Autodesk Fusion 360 part; units mm, degrees
sketch "Esquisse1" plane through (0, 0, 0) normal (0, 0, 1) x (1, 0, 0)
  line L0 (7, 0) -> (13, 0)
  line L1 (20, 7) -> (20, 21)
  line L2 (13, 28) -> (7, 28)
  line L3 (0, 21) -> (0, 7)
  line L4 (10, 28) -> (10, 0) construction
  circle A0 centre (10, 23.45) radius 2.1
  circle A1 centre (10, 4.55) radius 2.1
  line L5 (-6, 20) -> (25, 20) construction
  line L6 (25, 20) -> (25, 8) construction
  line L7 (25, 8) -> (-6, 8) construction
  line L8 (-6, 8) -> (-6, 20) construction
  line L9 (13, 0) -> (20, 7)
  line L10 (7, 0) -> (0, 7)
  line L11 (20, 21) -> (13, 28)
  line L12 (7, 28) -> (0, 21)
  point P0 (20, 0)
  point P1 (20, 28)
  point P2 (0, 28)
  dimension "d1" = 20
  dimension "d2" = 28
  dimension "d3" = 4.2
  dimension "d4" = 4.2
  dimension "d5" = 18.9
  dimension "d6" = 4.55
  dimension "d7" = 12
  dimension "d8" = 8
  dimension "d9" = 7
  dimension "d10" = 7
  dimension "d11" = 7
  dimension "d12" = 7
  dimension "d13" = 7
  dimension "d14" = 7
  dimension "d15" = 7
  dimension "d16" = 7
extrude "Extrusion1" add sketch "Esquisse1" along normal blind 14
sketch "Esquisse2" plane through (20, 0, 0) normal (1, 0, 0) x (0, 1, 0)
  line L0 (7, 0) -> (21, 0)
  line L1 (21, 0) -> (21, 14)
  line L2 (21, 14) -> (7, 14)
  line L3 (7, 14) -> (7, 0)
  circle A0 centre (14, 15) radius 6
  dimension "d19" = 12
  dimension "d20" = 15
  dimension "d21" = 7
extrude "Extrusion2" cut sketch "Esquisse2" against normal blind 20 contours L2 A0 | L2 A0
chamfer "Chanfrein1" distance 1.5 angle 45 8 edges at (16.5, 3.5, 0) (20, 14, 0) (16.5, 24.5, 0) (10, 28, 0) (3.5, 24.5, 0) (0, 14, 0) (3.5, 3.5, 0) (10, 0, 0)
fillet "Congé1" radius 0.5 22 edges at (10, 8.0839, 14) (10, 19.9161, 14) (0, 21, 7.75) (0, 7, 7.75) (0, 7.542, 14) (7, 0, 7.75) (13, 0, 7.75) (20, 7, 7.75) (20, 7.542, 14) (20, 14, 9) (0, 14, 9) (3.5, 24.5, 14) (10, 28, 14) (16.5, 24.5, 14) (20, 20.458, 14) (0, 20.458, 14) (20, 21, 7.75) (13, 28, 7.75) (7, 28, 7.75) (16.5, 3.5, 14) (10, 0, 14) (3.5, 3.5, 14)
fillet "Congé2" radius 0.5 8 edges at (0.769, 7.3185, 0.731) (7.3185, 0.769, 0.731) (12.6815, 0.769, 0.731) (0.769, 20.6815, 0.731) (7.3185, 27.231, 0.731) (12.6815, 27.231, 0.731) (19.231, 20.6815, 0.731) (19.231, 7.3185, 0.731)
equation "d5 = 14.7 mm + 4.2 mm"
equation "d6 = ( ( 28 - 18.9 ) / 2 ) * 1 mm"
equation "d10 = d9"
equation "d12 = d11"
equation "d14 = d13"
equation "d16 = d15"
The listing builds one solid part. Answer for the finished solid, in the listing's coordinates (mm). Round coordinates to 2 decimals unless told otherwise and drop trailing zeros. Order: outer loops, then holes, each group sorted by start corner. A loop starts at its lowest first (then second) coordinate and runs counter-clockwise, first axis right, second up. Notation, with made-up numbers: (19.5, -34.5) - (78.5, -34.5) arc R25 ccw to (78.5, -14.5) - close; hole circle Ø5 at (14.25, -6.75). An arc over 180 degrees is marked (long way). Write item = value, one per line. Start each with the question number.
1) Section C-C, the plane z = 10.75 is taken. Count the separate pieces of the cut face and the enclosed holes in it, plus the area to 3 significant figures.
2) Straight lines are drawn through the part: L1, parallel to Y at x = 10, z = 5.25; L2, parallel to X at y = 5.5, z = 13; L3, parallel to X at y = 6, z = 9.25. For each, find the intervals that lie inside material, in ascending order.
3) Section A-A, the plane z = 5.25 is taken. Write down the section's boundary in (x, y).
4) Given pin 1 (4 mm diameter, centred on x = 10, y = 4.55, fed in from +Z); pin 2 (1.5 mm diameter, centred on x = 12, y = 10, fed in from +Z); pin 3 (6 mm diameter, centred on x = 6.5, z = 8.5, fed in from +Y); pin 4 (5 mm diameter, centred on x = 16, y = 16, fed in from +Z), each flat-ended and moving along its own axis, determine where each tip first touches the part or whether it passes through.
5) Section B-B, the plane x = 10 is taken. Write down the section's boundary in (y, z), plus the area to 3 significant figures.
Results list:
q1.separate_pieces = 2
q1.enclosed_holes = 2
q1.area = 265 mm^2
q2.L1 = 0 to 2.45, 6.65 to 21.35, 25.55 to 28
q2.L2 = 1.5 to 8.13, 11.87 to 18.5
q2.L3 = 1 to 8.48, 11.52 to 19
q3.outline = (0, 7.21) arc R0.5 ccw to (0.15, 6.85) - (6.85, 0.15) arc R0.5 ccw to (7.21, 0) - (12.79, 0) arc R0.5 ccw to (13.15, 0.15) - (19.85, 6.85) arc R0.5 ccw to (20, 7.21) - (20, 20.79) arc R0.5 ccw to (19.85, 21.15) - (13.15, 27.85) arc R0.5 ccw to (12.79, 28) - (7.21, 28) arc R0.5 ccw to (6.85, 27.85) - (0.15, 21.15) arc R0.5 ccw to (0, 20.79) - close; hole circle Ø4.2 at (10, 4.55); hole circle Ø4.2 at (10, 23.45)
q4.pin_1 = through
q4.pin_2 = 11.33
q4.pin_3 = 28
q4.pin_4 = 11.03
q5.outline = (0, 1.5) - (1.5, 0) - (2.45, 0) - (2.45, 14) - (0.5, 14) arc R0.5 ccw to (0, 13.5) - close; (6.65, 0) - (21.35, 0) - (21.35, 14) - (20.32, 14) arc R0.5 ccw to (19.84, 13.62) arc R6 cw to (8.16, 13.62) arc R0.5 ccw to (7.68, 14) - (6.65, 14) - close; (25.55, 0) - (26.5, 0) - (28, 1.5) - (28, 13.5) arc R0.5 ccw to (27.5, 14) - (25.55, 14) - close
q5.area = 227 mm^2
